from build123d import *

# Parameters (mm, degrees)
EXTRUDE_1_DEPTH = 1.5
EXTRUDE_2_DEPTH = 0.5
SKETCH_3_R      = 0.75
EXTRUDE_3_DEPTH = 0.2


with BuildPart() as part:
    # 草图1 → 凸台-拉伸1 (new body)
    with BuildSketch(Plane.XY):
        with BuildLine():
            Line((7.3, 3.85), (-7.3, 3.85))
            ThreePointArc((-7.3, 3.85), (-11.15, 0), (-7.3, -3.85))
            Line((-7.3, -3.85), (7.3, -3.85))
            ThreePointArc((7.3, -3.85), (11.15, 0), (7.3, 3.85))
        make_face()
    extrude(amount=EXTRUDE_1_DEPTH)

    # 草图2 → 凸台-拉伸2 (add)
    with BuildSketch(Plane(origin=(0, 0, 0), x_dir=(-1, 0, 0), z_dir=(0, 0, -1))):
        with BuildLine():
            Line((-7.35, 2.3), (7.35, 2.3))
            ThreePointArc((7.35, 2.3), (9.65, 0), (7.35, -2.3))
            Line((7.35, -2.3), (-7.35, -2.3))
            ThreePointArc((-7.35, -2.3), (-9.65, 0), (-7.35, 2.3))
        make_face()
    extrude(amount=EXTRUDE_2_DEPTH)

    # 草图3 → 凸台-拉伸3 (add)
    with BuildSketch(Plane(origin=(0, 0, -0.5), x_dir=(-1, 0, 0), z_dir=(0, 0, -1))):
        with Locations((1.27, 0)):
            Circle(SKETCH_3_R)
        with Locations((3.81, 0)):
            Circle(SKETCH_3_R)
        with Locations((-3.81, 0)):
            Circle(SKETCH_3_R)
        with Locations((-1.27, 0)):
            Circle(SKETCH_3_R)
    extrude(amount=EXTRUDE_3_DEPTH)


solid = part.part
Input: part model. Units: mm. Frame: model coordinates. A direction names the side the tool comes from. Coordinates: 2 decimals unless noted, no trailing zeros. Order: outer loops, then holes, each group sorted by start corner. A loop starts at its lowest first (then second) coordinate and runs counter-clockwise, first axis right, second up. Notation, with made-up numbers: M 36.5,8.25 L 93.5,8.25 A9 ccw 93.5,19.25 Z; hole C -26,19.5 d11. An arc over 180 degrees is marked long. Answer in a Markdown table with one row per item.
(1) Material intervals for line 1 (Z direction, x = -7, y = 3); line 2 (Z direction, x = 9.25, y = -0.75); line 3 (Y direction, x = 7.5, z = 1.3), sorted ascending. Write a range as [from, to].
Numbers:
| item | result |
|---|---|
| line 1 | z = [0, 1.5] |
| line 2 | z = [-0.5, 1.5] |
| line 3 | y = [-3.84, 3.84] |
(2) Contact query for a flat-ended pin moving along its axis: pin 1 Ø4 at (x, y) = (-3, -1) entering from -Z. Output: stop coordinate, or through.
Numbers:
| item | result |
|---|---|
| pin 1 | stops at z = -0.7 |
(3) Section query A-A, the plane x = 7. Output: boundary loops of the cut face in (y, z), plus the area to 4 significant figures.
Numbers:
| item | result |
|---|---|
| outline | M -3.85,0 L -2.3,0 L -2.3,-0.5 L 2.3,-0.5 L 2.3,0 L 3.85,0 L 3.85,1.5 L -3.85,1.5 Z |
| area | 13.85 mm^2 |
(4) Section query C-C, the plane z = 0.3. Output: boundary loops of the cut face in (x, y).
Numbers:
| item | result |
|---|---|
| outline | M -7.3,-3.85 L 7.3,-3.85 A3.85 ccw 7.3,3.85 L -7.3,3.85 A3.85 ccw Z |
(5) Section query D-D, the plane x = 1.27. Output: boundary loops of the cut face in (y, z), plus the area to 4 significant figures.
Numbers:
| item | result |
|---|---|
| outline | M -3.85,0 L -2.3,0 L -2.3,-0.5 L -0.75,-0.5 L -0.75,-0.7 L 0.75,-0.7 L 0.75,-0.5 L 2.3,-0.5 L 2.3,0 L 3.85,0 L 3.85,1.5 L -3.85,1.5 Z |
| area | 14.15 mm^2 |
(6) Access query for faces 1 (the flat face through (0, -3.85, 1)), 2 (the cylindrical face through (9.65, -0.05, -0.25)), 3 (the flat face through (0, 0, -0.5)), 4 (the cylindrical face through (-9.65, 0.05, -0.25)), 5 (the flat face through (0, 3.85, 1)). Directions: +Z, -Z, +X, -X, +Y, -Y. A direction counts if a zero-diameter tool reaches every point of the face in a straight line with its end or side. Return the directions, or none.
Numbers:
| item | result |
|---|---|
| face 1 | +Z, -Z, +X, -X, -Y |
| face 2 | -Z, +X |
| face 3 | -Z |
| face 4 | -Z, -X |
| face 5 | +Z, -Z, +X, -X, +Y |
(7) Section query B-B, the plane y = 0. Output: boundary loops of the cut face in (x, z).
Numbers:
| item | result |
|---|---|
| outline | M -11.15,0 L -9.65,0 L -9.65,-0.5 L -4.56,-0.5 L -4.56,-0.7 L -3.06,-0.7 L -3.06,-0.5 L -2.02,-0.5 L -2.02,-0.7 L -0.52,-0.7 L -0.52,-0.5 L 0.52,-0.5 L 0.52,-0.7 L 2.02,-0.7 L 2.02,-0.5 L 3.06,-0.5 L 3.06,-0.7 L 4.56,-0.7 L 4.56,-0.5 L 9.65,-0.5 L 9.65,0 L 11.15,0 L 11.15,1.5 L -11.15,1.5 Z |
